Work out the finished part from the listing and answer in its coordinate system (mm). A direction names the side the tool comes from. Round coordinates to 2 decimals unless told otherwise and drop trailing zeros. Loops run counter-clockwise (first coordinate to the right, second up) from the corner with the lowest first, then second, coordinate; pieces in that order, holes last. Notation, with made-up numbers: (17.5, -14.75) - (65.5, -14.75) arc R10 cw to (65.5, -6.75) - close; hole circle Ø1 at (18, 55). An arc over 180 degrees is marked (long way). Answer as CSV lines item,"result". Start each with the question number.
Q1. Section B-B on x = -29 is taken. Write down the section's boundary in (y, z).
Q2. The mould has two halves that part along Y. Classify faces 1 (the face through (-38.1, -54.2, 52.1)), 2 (the face through (-38.127, -11.311, 81.706)), 3 (the face through (-38.057, -47.601, 56.146)): +Y half, -Y half, draft (parallel to the pull), parting line (faces both ways), or undercut.
Q3. Straight lines are drawn through the part: L1, parallel to X at y = -16.5, z = 32; L2, parallel to Y at x = -37, z = 12; L3, parallel to Y at x = -38, z = 40. For each, find the intervals that lie inside material, in ascending order. Write a range as [from, to].
Q4. Each of these flat-tipped pins is pushed along its axis until it touches: pin 1 Ø1.5 at (x, z) = (-39, 58.5) entering from +Y; pin 2 Ø3 at (x, z) = (-36.5, 26.5) entering from +Y; pin 3 Ø1.6 at (y, z) = (-14.5, 43) entering from +X. Where does it stop, or does it pass through?
Q5. For faces 4 (the face through (-38.057, -37.008, 13.399)), 5 (the face through (-38.127, 26.388, 58.298)), 6 (the face through (-31.14, -18.89, 42.35)), determine the directions among +Z, -Z, +X, -X, +Y, -Y from which every point of the face is accessible in a straight line to the end or side of a thin tool.
Q6. Section A-A on z = 15.5 is taken. Write down the section's boundary in (x, y), then the cut area to 3 significant figures.
Q7. Section D-D on z = 72 is taken. Write down the section's boundary in (x, y), then the cut area to 3 significant figures.
Q8. Section C-C on y = -23.5 is taken. Write down the section's boundary in (x, z), then the cut area to 3 significant figures.
```python
from build123d import *

# Parameters (mm, degrees)
EXTRUDE_2_DEPTH     = 2.5
SKETCH_4_R          = 6
EXTRUDE_3_DEPTH     = 8
CUT_EXTRUDE_5_DEPTH = 11.5
SKETCH_14_R         = 1.6
CUT_EXTRUDE_6_DEPTH = 12
SKETCH_15_R         = 1.3
CUT_EXTRUDE_7_DEPTH = 11
FILLET_7_R          = 1
FILLET1_R           = 3
SKETCH1_R           = 4
CUT_EXTRUDE2_DEPTH  = 50


with BuildPart() as part:
    # Sketch 2 → Extrude 2 (new, symmetric)
    with BuildSketch(Plane.ZY.offset(38.091621509)):
        with BuildLine():
            Line((50.911357014, 23.516558631), (55.24762265, 27.512579341))
            ThreePointArc((55.24762265, 27.512579341), (57.449397458, 26.727774506), (59.60469494, 25.823106776))
            ThreePointArc((59.60469494, 25.823106776), (55.850769285, 0.327394986), (79.444065843, -10.039843558))
            Line((79.444065843, -10.039843558), (84.584487152, -12.929038938))
            ThreePointArc((84.584487152, -12.929038938), (84.518479234, -15.265569248), (84.324112643, -17.594936665))
            ThreePointArc((84.324112643, -17.594936665), (58.916222984, -21.903349436), (56.347122801, -47.545560763))
            Line((56.347122801, -47.545560763), (55.187812251, -53.327202418))
            ThreePointArc((55.187812251, -53.327202418), (52.945242306, -53.986452731), (50.669819665, -54.521413236))
            ThreePointArc((50.669819665, -54.521413236), (38.720805929, -31.688446976), (13.539718137, -37.16896658))
            Line((13.539718137, -37.16896658), (7.682803504, -37.853022253))
            ThreePointArc((7.682803504, -37.853022253), (6.362826974, -35.923931044), (5.150905034, -33.925187402))
            ThreePointArc((5.150905034, -33.925187402), (23.173898072, -15.505225418), (10.180230126, 6.749838518))
            Line((10.180230126, 6.749838518), (7.719768364, 12.108710517))
            ThreePointArc((7.719768364, 12.108710517), (9.146547949, 13.960204765), (10.672961639, 15.730456776))
            ThreePointArc((10.672961639, 15.730456776), (33.760797652, 4.281653093), (50.911357014, 23.516558631))
        make_face()
    extrude(amount=EXTRUDE_2_DEPTH, both=True)

    # Sketch 4 → Extrude 3 (add)
    with BuildSketch(Plane(origin=(-35.591621509, 0, 0), x_dir=(0, 0, -1), z_dir=(1, 0, 0))):
        with Locations(Location((-42.084498784, -12.89759475, 0), (0, 0, 90))):
            Circle(SKETCH_4_R)
    extrude(amount=EXTRUDE_3_DEPTH)

    # Sketch 13 → Cut-Extrude 5 (cut)
    with BuildSketch(Plane(origin=(-27.591621509, 0, 0), x_dir=(0, 0, -1), z_dir=(1, 0, 0))):
        with BuildLine():
            Line((-44.364849634, -10.79759475), (-39.804147934, -10.79759475))
            ThreePointArc((-39.804147934, -10.79759475), (-42.084498784, -15.99759475), (-44.364849634, -10.79759475))
        make_face()
    extrude(amount=-CUT_EXTRUDE_5_DEPTH, mode=Mode.SUBTRACT)

    # Sketch 14 → Cut-Extrude 6 (cut)
    with BuildSketch(Plane.ZY.offset(40.591621509)):
        with Locations(Location((42.084498784, -12.89759475, 0), (0, 0, 270))):
            Circle(SKETCH_14_R)
    extrude(amount=-CUT_EXTRUDE_6_DEPTH, mode=Mode.SUBTRACT)

    # Sketch 15 → Cut-Extrude 7 (cut)
    with BuildSketch(Plane.XZ.offset(10.79759475)):
        with Locations((-31.591621509, 42.084498784)):
            Circle(SKETCH_15_R)
    extrude(amount=-CUT_EXTRUDE_7_DEPTH, mode=Mode.SUBTRACT)

    # Fillet 7
    fillet_7_edges = [part.edges().sort_by_distance(p)[0] for p in [
        (-35.591621509, -18.89759475, 42.084498784),
    ]]
    fillet(fillet_7_edges, radius=FILLET_7_R)

    # Fillet1
    fillet1_edges = [part.edges().sort_by_distance(p)[0] for p in [
        (-38.091621509, -37.853022253, 7.682803504),
        (-38.091621509, -37.16896658, 13.539718137),
        (-38.091621509, -53.327202418, 55.187812251),
        (-38.091621509, -47.545560763, 56.347122801),
        (-38.091621509, -12.929038938, 84.584487152),
        (-38.091621509, -10.039843558, 79.444065843),
        (-38.091621509, 27.512579341, 55.24762265),
        (-38.091621509, 23.516558631, 50.911357014),
        (-38.091621509, 12.108710517, 7.719768364),
        (-38.091621509, 6.749838518, 10.180230126),
    ]]
    fillet(fillet1_edges, radius=FILLET1_R)

    # Sketch1 → Cut-Extrude2 (cut)
    with BuildSketch(Plane.ZY.offset(40.591621509)):
        with Locations(Location((44.856906438, -3.289589973, 0), (0, 0, 270))):
            Circle(SKETCH1_R)
    extrude(amount=-CUT_EXTRUDE2_DEPTH, mode=Mode.SUBTRACT)


solid = part.part
```
Findings:
1,outline,"circle Ø12 at (-12.9, 42.08); hole (-10.8, 39.8) - (-10.8, 44.36) arc R3.1 ccw (long way) to start"
2,face 1,"-Y half"
2,face 2,"+Y half"
2,face 3,"undercut"
3,L1,"x = [-40.59, -35.59]"
3,L2,"y = [-37.35, -31.69], [5.9, 13.42]"
3,L3,"y = [-32.34, -15.19], [-10.8, 6.54]"
4,pin 1,"stops at y = 26.61"
4,pin 2,"stops at y = 4.43"
4,pin 3,"stops at x = -39.09"
5,face 4,"+X, -X, -Y"
5,face 5,"+Z, +X, -X, +Y"
5,face 6,"+X"
6,outline,"(-40.59, -35.15) - (-35.59, -35.15) - (-35.59, -29.38) - (-40.59, -29.38) - close; (-40.59, 3.58) - (-35.59, 3.58) - (-35.59, 9.36) - (-40.59, 9.36) - close"
6,area,"57.7 mm^2"
7,outline,"(-40.59, -15.3) - (-35.59, -15.3) - (-35.59, -10.5) - (-40.59, -10.5) - close"
7,area,"24.0 mm^2"
8,outline,"(-40.59, 20.5) - (-35.59, 20.5) - (-35.59, 57.57) - (-40.59, 57.57) - close"
8,area,"185 mm^2"
